Here's how the part is built. I have some questions about the finished solid (model axes, mm). A direction names the side the tool comes from. Coordinates: 2 decimals unless noted, no trailing zeros. Loops run counter-clockwise (first coordinate to the right, second up) from the corner with the lowest first, then second, coordinate; pieces in that order, holes last. Notation, with made-up numbers: (-35.75, -12) -> (18.25, -12) arc R20 ccw to (18.25, 6) -> close; hole circle Ø1 at (53.25, -12.5). An arc over 180 degrees is marked (long way). Answer as a JSON object with one key per item and string values. Group by question number.
Q1. I want a section at B-B on y = 8.5. Write out the boundary of the cut face in (x, z).
Q2. I need wall thicknesses on line 1 (X direction, y = 9.75, z = -2.25); line 2 (X direction, y = 9.5, z = -0.5); line 3 (Y direction, x = 0, z = 1). Which ranges of each line are inside material? Lowest first, please.
Q3. I want a section at A-A on x = 17.5. Write out the boundary of the cut face in (y, z).
Q4. Thinking about a two-plate mould opening in X: for faces 4 (the flat face through (39, 6, -1.5)), 5 (the flat face through (20.37, 3.5, 1.42)), 6 (the flat face through (-34.14, -1.95, 0.05)), which applies, released by +X, released by -X, zero draft, split by the parting line, or undercut?
Q5. I want a section at C-C on x = -11.5. Write out the boundary of the cut face in (y, z), then the cut area to 3 significant figures.
Q6. On a 3-axis mill with a long thin cutter (end or side, diameter ignored), from which of +Z, -Z, +X, -X, +Y, -Y can I reach the whole of each face in a straight line? I mean faces 1 (the flat face through (35, 4.6, -2)), 2 (the flat face through (17.831, 4.707, -0.76)), 3 (the flat face through (-21.5, 3, 1)). Say none if no direction works.
Q7. I'm going to push flat-ended pins straight in: pin 1 (0.8 mm diameter, centred on x = 34.5, z = -1.5, fed in from -Y); pin 2 (2 mm diameter, centred on y = 8, z = 1.5, fed in from +X); pin 3 (3 mm diameter, centred on y = 7.5, z = -1.5, fed in from +X); pin 4 (2 mm diameter, centred on x = -35.5, z = 2.5, fed in from -Y). Where does each tip first touch, or does it pass through?
Q8. I want a section at D-D on x = 31.5. Write out the boundary of the cut face in (y, z).
```python
from build123d import *

# Parameters (mm, degrees)
SKETCH1_W               = 2.8
SKETCH1_H               = 2.8
BOSS_EXTRUDE1_DEPTH     = 3.5
CUT_EXTRUDE1_DEPTH      = 42
CUT_EXTRUDE1_DEPTH_BACK = 42
CUT_EXTRUDE2_DEPTH      = 2.3
FILLET1_R               = 2
FILLET2_R               = 5
FILLET3_R               = 1


with BuildPart() as part:
    # Sketch1 → Boss-Extrude1 (new body, symmetric)
    with BuildSketch(Plane.XY):
        with BuildLine():
            Line((16.5, 0), (-16.5, 0))
            Line((-16.5, 0), (-16.5, 12))
            Line((-16.5, 12), (-21.5, 12))
            Line((-21.5, 12), (-21.5, 0))
            Line((-21.5, 0), (-26.5, 0))
            Line((-26.5, 0), (-26.5, 12))
            Line((-26.5, 12), (-35, 12))
            ThreePointArc((-35, 12), (-40.718865407, 7.81509737), (-38.460099186, 1.09819282))
            Line((-38.460099186, 1.09819282), (-28.404326023, -6))
            Line((-28.404326023, -6), (28.404326023, -6))
            Line((28.404326023, -6), (38.460099186, 1.09819282))
            ThreePointArc((38.460099186, 1.09819282), (40.718865407, 7.81509737), (35, 12))
            Line((35, 12), (26.5, 12))
            Line((26.5, 12), (26.5, 0))
            Line((26.5, 0), (21.5, 0))
            Line((21.5, 0), (21.5, 12))
            Line((21.5, 12), (16.5, 12))
            Line((16.5, 12), (16.5, 0))
        make_face()
        with Locations((35, 6)):
            Rectangle(SKETCH1_W, SKETCH1_H, mode=Mode.SUBTRACT)
        with Locations((-35, 6)):
            Rectangle(SKETCH1_W, SKETCH1_H, mode=Mode.SUBTRACT)
    extrude(amount=BOSS_EXTRUDE1_DEPTH, both=True)

    # Sketch2 → Cut-Extrude1 (cut, two sides)
    with BuildSketch(Plane.ZY) as cut_extrude1_sk:
        Polygon((0, 7.732050808), (-1.5, 6.866025404), (-1.5, 5.133974596), (0, 4.267949192), (1.5, 5.133974596), (1.5, 6.866025404), align=None)
    extrude(amount=CUT_EXTRUDE1_DEPTH, mode=Mode.SUBTRACT)
    extrude(cut_extrude1_sk.sketch, amount=-CUT_EXTRUDE1_DEPTH_BACK, mode=Mode.SUBTRACT)

    # Sketch3 → Cut-Extrude2 (cut)
    with BuildSketch(Plane.ZY.offset(21.5)):
        Polygon((2.875, 7.659882024), (0, 9.319764048), (-2.875, 7.659882024), (-2.875, 4.340117976), (0, 2.680235952), (2.875, 4.340117976), align=None)
    cut_extrude2 = extrude(amount=-CUT_EXTRUDE2_DEPTH, mode=Mode.SUBTRACT)

    # Mirror1: Cut-Extrude2 across plane
    add(cut_extrude2.mirror(Plane(origin=(0, 0, 0), x_dir=(0, 0, 1), z_dir=(1, 0, 0))), mode=Mode.SUBTRACT)

    # Fillet1
    fillet1_edges = [part.edges().sort_by_distance(p)[0] for p in [
        (-16.5, 12, 0),
        (-16.5, 0, 0),
        (16.5, 0, 0),
        (16.5, 12, 0),
        (21.5, 12, 0),
        (26.5, 12, 0),
        (-26.5, 12, 0),
        (-21.5, 12, 0),
    ]]
    fillet(fillet1_edges, radius=FILLET1_R)

    # Fillet2
    fillet2_edges = [part.edges().sort_by_distance(p)[0] for p in [
        (28.404326023, -6, 0),
        (-28.404326023, -6, 0),
    ]]
    fillet(fillet2_edges, radius=FILLET2_R)

    # Fillet3
    fillet3_edges = [part.edges().sort_by_distance(p)[0] for p in [
        (21.5, 0, 0),
        (26.5, 0, 0),
        (-26.5, 0, 0),
        (-21.5, 0, 0),
    ]]
    fillet(fillet3_edges, radius=FILLET3_R)


solid = part.part
```
Result set:
{
 "1": {"outline": "(-40.45, -3.5) -> (-26.5, -3.5) -> (-26.5, 3.5) -> (-40.45, 3.5) -> close; (-21.5, -3.5) -> (-16.5, -3.5) -> (-16.5, 3.5) -> (-21.5, 3.5) -> (-21.5, 1.42) -> (-19.2, 1.42) -> (-19.2, -1.42) -> (-21.5, -1.42) -> close; (16.5, -3.5) -> (21.5, -3.5) -> (21.5, -1.42) -> (19.2, -1.42) -> (19.2, 1.42) -> (21.5, 1.42) -> (21.5, 3.5) -> (16.5, 3.5) -> close; (26.5, -3.5) -> (40.45, -3.5) -> (40.45, 3.5) -> (26.5, 3.5) -> close"},
 "2": {"line 1": "x = -39.68 to -26.5, -21.5 to -16.5, 16.5 to 21.5, 26.5 to 39.68", "line 2": "x = -39.87 to -26.5, -21.5 to -16.5, 16.5 to 21.5, 26.5 to 39.87", "line 3": "y = -6 to 0"},
 "3": {"outline": "(-6, -3.5) -> (11.73, -3.5) -> (11.73, 3.5) -> (-6, 3.5) -> close; hole (4.27, 0) -> (5.13, -1.5) -> (6.87, -1.5) -> (7.73, 0) -> (6.87, 1.5) -> (5.13, 1.5) -> close"},
 "4": {"face 4": "zero draft", "face 5": "undercut", "face 6": "released by -X"},
 "5": {"outline": "(-6, -3.5) -> (0, -3.5) -> (0, 3.5) -> (-6, 3.5) -> close", "area": "42.0 mm²"},
 "6": {"face 1": "+Z, -Z", "face 2": "+X, -X", "face 3": "+Z, -Z, +Y"},
 "7": {"pin 1": "stops at y = -1.98", "pin 2": "stops at x = 40.92", "pin 3": "stops at x = 41", "pin 4": "stops at y = -1.7"},
 "8": {"outline": "(-3.81, -3.5) -> (12, -3.5) -> (12, 3.5) -> (-3.81, 3.5) -> close; hole (4.27, 0) -> (5.13, -1.5) -> (6.87, -1.5) -> (7.73, 0) -> (6.87, 1.5) -> (5.13, 1.5) -> close"}
}
